Check sheet for the drawn part. Datum: minimum x, y, z corner. Units: mm. Round coordinates to 2 decimals unless told otherwise and drop trailing zeros. Order: outer loops, then holes, each group sorted by start corner. A loop starts at its lowest first (then second) coordinate and runs counter-clockwise, first axis right, second up. Notation, with made-up numbers: (41, 71.25) -> (69, 71.25) arc R25 ccw to (69, 89.25) -> close; hole circle Ø2 at (75.25, 56). An arc over 180 degrees is marked (long way). Answer as a JSON object with one key per item and string values. Group by question number.
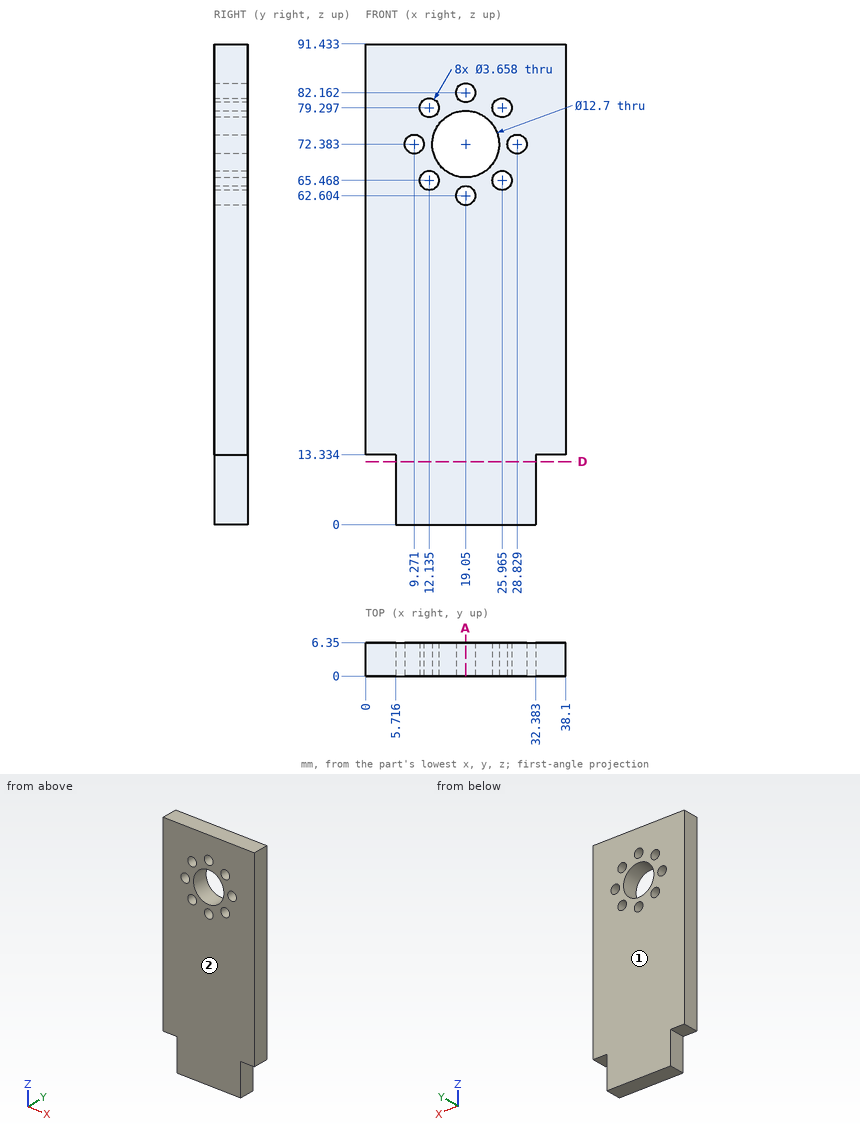
Item 1: Sectioned sample at A-A, the plane x = 19.05. Count the separate pieces of the cut face and the enclosed holes in it.
Item 2: Mould release check, pull along Y, two halves, no side actions. Record for the marked faces 1 and 2: pulls with the +Y half, pulls with the -Y half, needs draft (parallel to the pull), parting line crosses it, or undercut.
Item 3: Depth check by flat-ended pin: pin 1 Ø1.9 at (y, z) = (4, 7.5) entering from -X; pin 2 Ø1 at (y, z) = (4, 10) entering from +X. Enter the tip coordinate at first touch or a pass-through.
Item 4: Thickness scan on L1, parallel to X at y = 6, z = 73; L2, parallel to X at y = 1.25, z = 83.5 (1 decimal); L3, parallel to Z at x = 28.5, y = 1.5. Record the ranges inside material, lowest first.
Item 5: Sectioned sample at D-D, the plane z = 12. Enter the section's corners in (x, y), then the cut area to 3 significant figures.
Result:
{
 "1": {"separate pieces": "4", "enclosed holes": "0"},
 "2": {"face 1": "pulls with the +Y half", "face 2": "pulls with the -Y half"},
 "3": {"pin 1": "stops at x = 5.72", "pin 2": "stops at x = 32.38"},
 "4": {"L1": "x = 0 to 7.55, 10.99 to 12.73, 25.37 to 27.11, 30.55 to 38.1", "L2": "x = 0 to 17.8, 20.3 to 38.1", "L3": "z = 0 to 70.58, 74.18 to 91.43"},
 "5": {"outline": "(5.72, 0) -> (32.38, 0) -> (32.38, 6.35) -> (5.72, 6.35) -> close", "area": "169 mm2"}
}
